from build123d import *

# Parameters (mm, degrees)
ESQUISSE2_R                = 1.6
FIXINGHOLE_DEPTH           = 9.5
FIXINGHOLEREPETITION_COUNT = 4


with BuildPart() as part:
    # Esquisse1 → MainRevolution (revolve)
    with BuildSketch(Plane.XY):
        Polygon((11, 8.5), (11, 3), (0, 3), (0, 0), (16, 0), (16, 8.5), align=None)
    revolve(axis=Axis((0, 8.4, 0), (0, -1, 0)))

    # Esquisse2 → FixingHole (cut, through all)
    with BuildSketch(Plane(origin=(0, 8.5, 0), x_dir=(1, 0, 0), z_dir=(0, 1, 0))):
        with Locations((13.5, 0)):
            Circle(ESQUISSE2_R)
    fixinghole = extrude(amount=-FIXINGHOLE_DEPTH, mode=Mode.SUBTRACT)

    # FixingHoleRepetition: FixingHole ×4 about axis
    fixingholerepetition_axis = Axis((0, 0, 0), (0, 1, 0))
    for i in range(1, FIXINGHOLEREPETITION_COUNT):
        add(fixinghole.rotate(fixingholerepetition_axis, i * 360 / FIXINGHOLEREPETITION_COUNT), mode=Mode.SUBTRACT)


solid = part.part
Model file for the job. Use its own axes, mm. A direction names the side the tool comes from. Round coordinates to 2 decimals unless told otherwise and drop trailing zeros. Loops run counter-clockwise (first coordinate to the right, second up) from the corner with the lowest first, then second, coordinate; pieces in that order, holes last.
1. Band-saw the part on D-D, the plane x = -13.5. List the corners of the cut face in (y, z), and give its area (3 significant figures).
Check values:
outline: (0, -8.59) - (8.5, -8.59) - (8.5, -1.6) - (0, -1.6) - close; (0, 1.6) - (8.5, 1.6) - (8.5, 8.59) - (0, 8.59) - close
area: 119 mm2
2. Wall check: probe 1 along Z at (x, y) = (1, 5); probe 2 along X at (y, z) = (8, -6). Give the ranges that are in metal, low to high.
Check values:
probe 1: z = -15.97 to -14.75, -12.25 to -10.95, 10.95 to 12.25, 14.75 to 15.97
probe 2: x = -14.83 to -9.22, 9.22 to 14.83
3. Band-saw the part on C-C, the plane z = 0. List the corners of the cut face in (x, y).
Check values:
outline: (-16, 0) - (-15.1, 0) - (-15.1, 8.5) - (-16, 8.5) - close; (-11.9, 0) - (11.9, 0) - (11.9, 8.5) - (11, 8.5) - (11, 3) - (-11, 3) - (-11, 8.5) - (-11.9, 8.5) - close; (15.1, 0) - (16, 0) - (16, 8.5) - (15.1, 8.5) - close
4. Tool access for faces 5 (the cylindrical face through (0.07, 4.31, 11.9)), 6 (the cylindrical face through (-2.38, 5.71, -10.74)): list every direction of +Z, -Z, +X, -X, +Y, -Y with a clear straight run to the whole face (end or side of a thin tool).
Check values:
face 5: +Y, -Y
face 6: +Y
5. Band-saw the part on B-B, the plane y = 2. List the corners of the cut face in (x, z), and give its area (3 significant figures).
Check values:
outline: circle Ø32 at (0, 0); hole circle Ø3.2 at (-13.5, 0); hole circle Ø3.2 at (0, -13.5); hole circle Ø3.2 at (0, 13.5); hole circle Ø3.2 at (13.5, 0)
area: 772 mm2
6. Mould opens along Z. For faces 1 (the cylindrical face through (-0.07, 4.31, -11.9)), 2 (the cylindrical face through (-3.47, 4.31, -15.62)), 3 (the cylindrical face through (11.9, 4.31, -0.07)), 4 (the flat face through (0, 0, 0)) say: +Z half, -Z half, draft (parallel to the pull), parting line (faces both ways), or undercut.
Check values:
face 1: undercut
face 2: parting line
face 3: undercut
face 4: draft
7. Drop flat-ended pins along their axis: P1, Ø12, axis at x = -2, z = 1.5, coming from the -Y side; P2, Ø3, axis at y = 1.5, z = 11.5, coming from the -X side; P3, Ø5, axis at x = -5, y = 7, coming from the +Z side; P4, Ø3, axis at x = 3, y = 3, coming from the +Z side. Give the stop position or say it passes through.
Check values:
P1: stops at y = 0
P2: stops at x = -12.49
P3: stops at z = 15.8
P4: stops at z = 15.93
8. Band-saw the part on A-A, the plane x = 0. List the corners of the cut face in (y, z).
Check values:
outline: (0, -16) - (8.5, -16) - (8.5, -15.1) - (0, -15.1) - close; (0, -11.9) - (8.5, -11.9) - (8.5, -11) - (3, -11) - (3, 11) - (8.5, 11) - (8.5, 11.9) - (0, 11.9) - close; (0, 15.1) - (8.5, 15.1) - (8.5, 16) - (0, 16) - close
